For this review, take the finished solid that the model builds, in its own axes (mm). Round coordinates to 2 decimals unless told otherwise and drop trailing zeros. Order: outer loops, then holes, each group sorted by start corner. A loop starts at its lowest first (then second) coordinate and runs counter-clockwise, first axis right, second up.
```python
from build123d import *

# Parameters (mm, degrees)
SKETCH_R  = 1.375
PAD_DEPTH = 3


with BuildPart() as part:
    # Sketch → Pad (new body)
    with BuildSketch(Plane.XY):
        with BuildLine():
            ThreePointArc((0, 2.12132), (0.62132, 0.62132), (2.12132, 0))
            Line((82.87868, 0), (2.12132, 0))
            ThreePointArc((82.87868, 0), (84.37868, 0.62132), (85, 2.12132))
            Line((85, 53.87868), (85, 2.12132))
            ThreePointArc((85, 53.87868), (84.37868, 55.37868), (82.87868, 56))
            Line((2.12132, 56), (82.87868, 56))
            ThreePointArc((2.12132, 56), (0.62132, 55.37868), (0, 53.87868))
            Line((0, 2.12132), (0, 53.87868))
        make_face()
        with Locations((3.5, 3.5)):
            Circle(SKETCH_R, mode=Mode.SUBTRACT)
        with Locations((3.5, 52.5)):
            Circle(SKETCH_R, mode=Mode.SUBTRACT)
        with Locations((58, 52.5)):
            Circle(SKETCH_R, mode=Mode.SUBTRACT)
        with Locations((58, 3.5)):
            Circle(SKETCH_R, mode=Mode.SUBTRACT)
    extrude(amount=PAD_DEPTH)


solid = part.part
```
Q1. Mouldability with a two-part tool opening along Y and no side actions: class faces 1 (the face through (0.638, 55.395, 1.479)), 2 (the face through (43, 0, 1)), 3 (the face through (57.7, 51.16, 1.48)), 4 (the face through (4.77, 2.97, 1.48)) as +Y half, -Y half, draft (parallel to the pull), parting line (faces both ways), or undercut.
Q2. Take a section at B-B, the plane x = 58. State the section outline as (y, z) points (3 decimals).
Q3. Take a section at A-A, the plane y = 3.5. State the section outline as (x, z) points (3 decimals).
Q4. Wall thickness on line 1 (Y direction, x = 58, z = 1) (3 decimals); line 2 (X direction, y = 4, z = 0.5): over which ranges is each line inside the solid? List them lowest first.
Q5. Clearance check with a flat-ended pin moving along its axis: pin 1 (2 mm diameter, centred on x = 3.5, y = 52.5, fed in from +Z). State where the tip first meets the part, or that it passes through.
Working result:
1. face 1: +Y half
1. face 2: -Y half
1. face 3: undercut
1. face 4: undercut
2. outline: (0, 0) - (2.125, 0) - (2.125, 3) - (0, 3) - close; (4.875, 0) - (51.125, 0) - (51.125, 3) - (4.875, 3) - close; (53.875, 0) - (56, 0) - (56, 3) - (53.875, 3) - close
3. outline: (0, 0) - (2.125, 0) - (2.125, 3) - (0, 3) - close; (4.875, 0) - (56.625, 0) - (56.625, 3) - (4.875, 3) - close; (59.375, 0) - (85, 0) - (85, 3) - (59.375, 3) - close
4. line 1: y = 0 to 2.125, 4.875 to 51.125, 53.875 to 56
4. line 2: x = 0 to 2.22, 4.78 to 56.72, 59.28 to 85
5. pin 1: passes through
